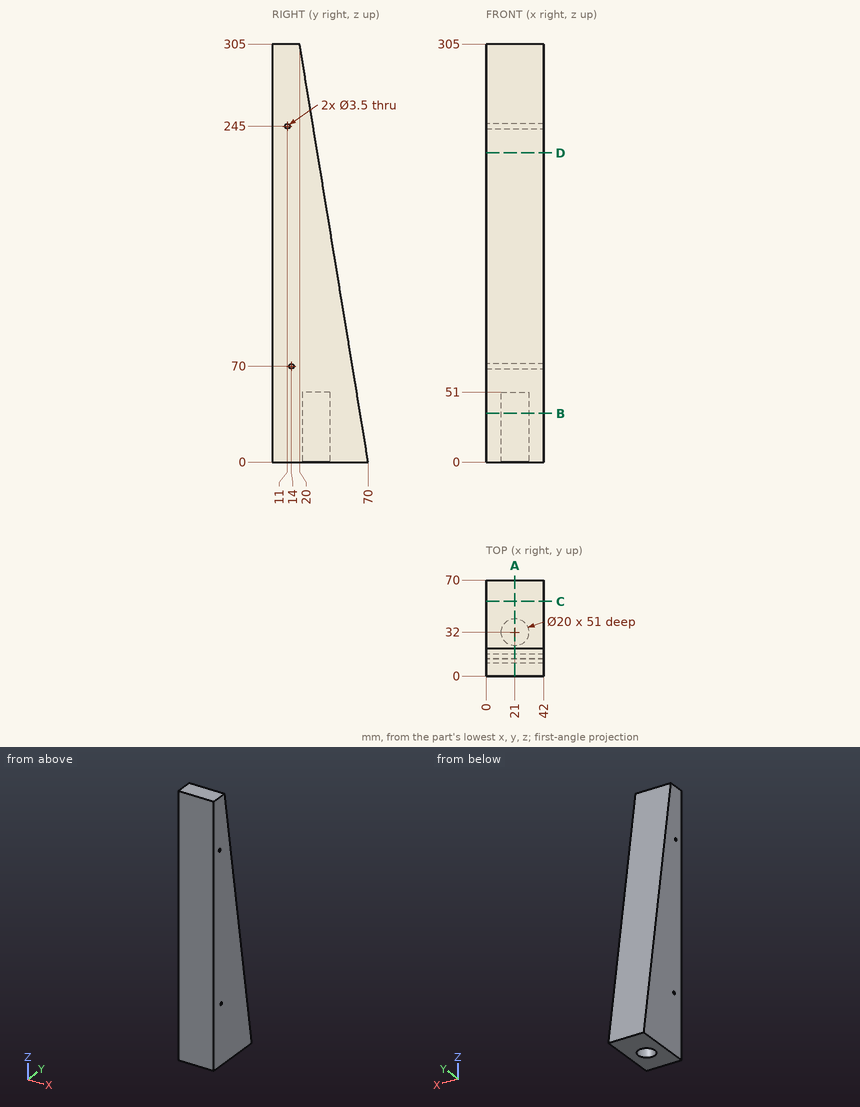
The drawing under review shows one solid part. Ordinate dimensions are in mm from its lowest x, y, z. Coordinates: 2 decimals unless noted, no trailing zeros. Order: outer loops, then holes, each group sorted by start corner. A loop starts at its lowest first (then second) coordinate and runs counter-clockwise, first axis right, second up. Notation, with made-up numbers: M -2.75,-12.5 L 7.25,-12.5 A20 ccw 7.25,6.5 Z; hole C 48.5,25.5 d4. An arc over 180 degrees is marked long. Use a Markdown table: item, result.
(1) Add section B-B (z = 35.5). Give the boundary of the cut face in (x, y), then the cut area to 3 significant figures.
Worked answers:
| item | result |
|---|---|
| outline | M 0,0 L 42,0 L 42,64.18 L 0,64.18 Z; hole C 21,32 d20 |
| area | 2,380 mm2 |
(2) Wall thickness on probe 1 along Z at (x, y) = (18, 14); probe 2 along Y at (x, z) = (13, 245); probe 3 along Z at (x, y) = (35, 10): over which ranges is each line inside the solid? List them lowest first.
Worked answers:
| item | result |
|---|---|
| probe 1 | z = 0 to 68.25, 71.75 to 305 |
| probe 2 | y = 0 to 9.25, 12.75 to 29.84 |
| probe 3 | z = 0 to 243.56, 246.44 to 305 |
(3) Add section C-C (y = 54.5). Give the boundary of the cut face in (x, z), then the cut area to 3 significant figures.
Worked answers:
| item | result |
|---|---|
| outline | M 0,0 L 42,0 L 42,94.55 L 0,94.55 Z |
| area | 3,970 mm2 |
(4) Add section D-D (z = 225.5). Give the boundary of the cut face in (x, y), then the cut area to 3 significant figures.
Worked answers:
| item | result |
|---|---|
| outline | M 0,0 L 42,0 L 42,33.03 L 0,33.03 Z |
| area | 1,390 mm2 |
(5) Add section A-A (x = 21). Give the boundary of the cut face in (y, z), then the cut area to 3 significant figures.
Worked answers:
| item | result |
|---|---|
| outline | M 0,0 L 22,0 L 22,51 L 42,51 L 42,0 L 70,0 L 20,305 L 0,305 Z; hole C 11,245 d3.5; hole C 14,70 d3.5 |
| area | 12,700 mm2 |
(6) For P1, Ø10, axis at x = 23, y = 31, coming from the -Z side; P2, Ø3, axis at y = 11, z = 245, coming from the -X side; P3, Ø1.5, axis at x = 11, z = 207, coming from the +Y side; P4, Ø1, axis at x = 27.5, z = 142, coming from the +Y side, all flat-tipped, find the tip position at first contact; note any pin that passes through.
Worked answers:
| item | result |
|---|---|
| P1 | stops at z = 51 |
| P2 | passes through |
| P3 | stops at y = 36.19 |
| P4 | stops at y = 46.8 |
